Input: part model. Units: mm. Frame: model coordinates. A direction names the side the tool comes from. Coordinates: 2 decimals unless noted, no trailing zeros. Write each loop counter-clockwise with the first axis right and the second up, starting at its lowest first coordinate (ties: lowest second). Pieces come first, ordered by that corner, then holes. Notation, with made-up numbers: (86, 40) - (107, 40) arc R20 cw to (107, 56) - close; hole circle Ø5 at (14.25, 25.5). An arc over 180 degrees is marked (long way). Use a Markdown table: item, result. Add a question column.
Q1. Section query B-B (y = 6). Return the cut outline in (x, z).
Q2. Material intervals for probe 1 along X at (y, z) = (5.75, -20.75); probe 2 along X at (y, z) = (1.25, -30.5); probe 3 along Z at (x, y) = (-8.5, 2.75), sorted ascending. Write a range as from..to.
Q3. Section query C-C (x = -8.75). Return the cut outline in (y, z).
Q4. Section query A-A (y = 1.75). Return the cut outline in (x, z), then the cut area to 3 significant figures.
Q5. Set-up query: faces 4 (the face through (-17.374, 5, -23)), 5 (the face through (-8, 6, -27.659)), 6 (the face through (-9.974, 5, -34)). Return all of +Z, -Z, +X, -X, +Y, -Y with unobstructed straight access to the full face (end or side cutting, diameter ignored); none if empty.
Q6. Mould query, pull axis X, two halves, no side actions, for faces 1 (the face through (-14, 7, -37.159)), 2 (the face through (-17.374, 5, -34)), 3 (the face through (-13.6, 3.7, -27.7)). Classes: released by +X, released by -X, zero draft, split by the parting line, or undercut.
Q7. Section query D-D (z = -23.25). Return the cut outline in (x, y), then the cut area to 3 significant figures.
Q8. Pin query (flat end, axial travel): P1, Ø1.3, axis at x = -20.5, y = 3, coming from the +Z side; P2, Ø3, axis at y = 5, z = -22.5, coming from the -X side; P3, Ø2, axis at x = -7.5, y = 7.5, coming from the -Z side. Return the tip coordinate at first contact, or that it passes through.
from build123d import *

# Parameters (mm, degrees)
BOSS_EXTRU_1_DEPTH      = 11
ENL_V_MAT_EXTRU_1_DEPTH = 31.697565104
ESQUISSE3_W             = 4.3
ESQUISSE3_H             = 0.5
ENL_V_MAT_EXTRU_2_DEPTH = 45.402774751


with BuildPart() as part:
    # Esquisse1 → Boss.-Extru.1 (new body)
    with BuildSketch(Plane(origin=(0, 0, 0), x_dir=(1, 0, 0), z_dir=(0, 1, 0))):
        Polygon((-17.374362812, 37.159499489), (-9.974362812, 37.159499489), (-9.974362812, 32.159499489), (-5.674362812, 32.159499489), (-5.674362812, 27.159499489), (-9.974362812, 27.159499489), (-9.974362812, 18.409499489), (-17.374362812, 18.409499489), (-17.374362812, 27.159499489), (-21.674362812, 27.159499489), (-21.674362812, 32.159499489), (-17.374362812, 32.159499489), align=None)
    extrude(amount=BOSS_EXTRU_1_DEPTH)

    # Esquisse2 → Enlèv. mat.-Extru.1 (cut, through all)
    with BuildSketch(Plane.XY.offset(-18.409499489)):
        with BuildLine():
            ThreePointArc((-9.974362812, 0), (-13.674362812, 3.7), (-17.374362812, 0))
            Line((-17.374362812, 0), (-9.974362812, 0))
        make_face()
        with BuildLine():
            Line((-9.974362812, 0), (-17.374362812, 0))
            ThreePointArc((-17.374362812, 0), (-13.674362812, -3.7), (-9.974362812, 0))
        make_face()
    extrude(amount=-ENL_V_MAT_EXTRU_1_DEPTH, mode=Mode.SUBTRACT)

    # Esquisse3 → Enlèv. mat.-Extru.2 (cut, through all)
    with BuildSketch(Plane(origin=(0, 11, 0), x_dir=(1, 0, 0), z_dir=(0, 1, 0))):
        with Locations((-7.824362812, 31.909499489)):
            Rectangle(ESQUISSE3_W, ESQUISSE3_H)
        with Locations((-19.524362812, 31.909499489)):
            Rectangle(ESQUISSE3_W, ESQUISSE3_H)
        with Locations((-19.524362812, 27.409499489)):
            Rectangle(ESQUISSE3_W, ESQUISSE3_H)
        with Locations((-7.824362812, 27.409499489)):
            Rectangle(ESQUISSE3_W, ESQUISSE3_H)
    extrude(amount=-ENL_V_MAT_EXTRU_2_DEPTH, mode=Mode.SUBTRACT)


solid = part.part
Values follow:
| question | item | result |
|---|---|---|
| 1 | outline | (-21.67, -31.66) - (-17.37, -31.66) - (-17.37, -37.16) - (-9.97, -37.16) - (-9.97, -31.66) - (-5.67, -31.66) - (-5.67, -27.66) - (-9.97, -27.66) - (-9.97, -18.41) - (-17.37, -18.41) - (-17.37, -27.66) - (-21.67, -27.66) - close |
| 2 | probe 1 | -17.37..-9.97 |
| 2 | probe 2 | -21.67..-17.16, -10.19..-5.67 |
| 2 | probe 3 | -31.66..-27.66 |
| 3 | outline | (0, -31.66) - (11, -31.66) - (11, -27.66) - (0, -27.66) - close |
| 4 | outline | (-21.67, -31.66) - (-17.37, -31.66) - (-17.37, -37.16) - (-16.93, -37.16) - (-16.93, -18.41) - (-17.37, -18.41) - (-17.37, -27.66) - (-21.67, -27.66) - close; (-10.41, -37.16) - (-9.97, -37.16) - (-9.97, -31.66) - (-5.67, -31.66) - (-5.67, -27.66) - (-9.97, -27.66) - (-9.97, -18.41) - (-10.41, -18.41) - close |
| 4 | area | 50.9 mm2 |
| 5 | face 4 | +Z, -X, +Y, -Y |
| 5 | face 5 | +Z, +X, +Y, -Y |
| 5 | face 6 | -Z, +X, +Y, -Y |
| 6 | face 1 | zero draft |
| 6 | face 2 | released by -X |
| 6 | face 3 | undercut |
| 7 | outline | (-17.37, 0) arc R3.7 cw to (-9.97, 0) - (-9.97, 11) - (-17.37, 11) - close |
| 7 | area | 59.9 mm2 |
| 8 | P1 | z = -27.66 |
| 8 | P2 | x = -17.37 |
| 8 | P3 | z = -31.66 |
